Can you work these out from the model? Positions are in its coordinate system, mm. A direction names the side the tool comes from. Coordinates: 2 decimals unless noted, no trailing zeros. Order: outer loops, then holes, each group sorted by start corner. A loop starts at its lowest first (then second) coordinate and runs counter-clockwise, first axis right, second up. Notation, with made-up numbers: (47.5, 88.5) -> (100.5, 88.5) arc R26 ccw to (100.5, 107.5) -> close; hole circle Ø10 at (40.25, 72). An arc over 180 degrees is marked (long way). Write item = value, one per line.
```python
from build123d import *

# Parameters (mm, degrees)
SKETCH_1_W          = 200
SKETCH_1_H          = 400
EXTRUDE_1_DEPTH     = 8
SKETCH_2_R          = 30
CUT_EXTRUDE_1_DEPTH = 10
SKETCH_3_R          = 2.25
CUT_EXTRUDE_2_DEPTH = 10
SKETCH_4_R          = 4
CUT_EXTRUDE_3_DEPTH = 4.4
FILLET_1_R          = 60
SKETCH_5_R          = 4.25
CUT_EXTRUDE_4_DEPTH = 10
SKETCH_6_W          = 50
SKETCH_6_H          = 220
CUT_EXTRUDE_5_DEPTH = 10
FILLET_2_R          = 10
SKETCH_7_W          = 100
SKETCH_7_H          = 120
CUT_EXTRUDE_6_DEPTH = 84
FILLET_3_R          = 10


with BuildPart() as part:
    # 草图1 → 凸台-拉伸1 (new body)
    with BuildSketch(Plane.XY):
        with Locations((0, 200)):
            Rectangle(SKETCH_1_W, SKETCH_1_H)
    extrude(amount=EXTRUDE_1_DEPTH)

    # 草图2 → 切除-拉伸1 (cut)
    with BuildSketch(Plane(origin=(0, 0, 0), x_dir=(-1, 0, 0), z_dir=(0, 0, -1))):
        with Locations((0, 300)):
            Circle(SKETCH_2_R)
    extrude(amount=-CUT_EXTRUDE_1_DEPTH, mode=Mode.SUBTRACT)

    # 草图3 → 切除-拉伸2 (cut)
    with BuildSketch(Plane(origin=(0, 0, 0), x_dir=(-1, 0, 0), z_dir=(0, 0, -1))):
        with Locations((0, 341.5)):
            Circle(SKETCH_3_R)
        with Locations((29.344931419, 329.344931419)):
            Circle(SKETCH_3_R)
        with Locations((41.5, 300)):
            Circle(SKETCH_3_R)
        with Locations((29.344931419, 270.655068581)):
            Circle(SKETCH_3_R)
        with Locations((0, 258.5)):
            Circle(SKETCH_3_R)
        with Locations((-29.344931419, 270.655068581)):
            Circle(SKETCH_3_R)
        with Locations((-41.5, 300)):
            Circle(SKETCH_3_R)
        with Locations((-29.344931419, 329.344931419)):
            Circle(SKETCH_3_R)
    extrude(amount=-CUT_EXTRUDE_2_DEPTH, mode=Mode.SUBTRACT)

    # 草图4 → 切除-拉伸3 (cut)
    with BuildSketch(Plane.XY.offset(8)):
        with Locations((29.344931419, 329.344931419)):
            Circle(SKETCH_4_R)
        with Locations((41.5, 300)):
            Circle(SKETCH_4_R)
        with Locations((29.344931419, 270.655068581)):
            Circle(SKETCH_4_R)
        with Locations((0, 258.5)):
            Circle(SKETCH_4_R)
        with Locations((-29.344931419, 270.655068581)):
            Circle(SKETCH_4_R)
        with Locations((-41.5, 300)):
            Circle(SKETCH_4_R)
        with Locations((-29.344931419, 329.344931419)):
            Circle(SKETCH_4_R)
        with Locations((0, 341.5)):
            Circle(SKETCH_4_R)
    extrude(amount=-CUT_EXTRUDE_3_DEPTH, mode=Mode.SUBTRACT)

    # 圆角1
    fillet_1_edges = [part.edges().sort_by_distance(p)[0] for p in [
        (100, 400, 4),
        (-100, 400, 4),
    ]]
    fillet(fillet_1_edges, radius=FILLET_1_R)

    # 草图5 → 切除-拉伸4 (cut)
    with BuildSketch(Plane(origin=(0, 0, 0), x_dir=(-1, 0, 0), z_dir=(0, 0, -1))):
        with Locations((-15, 25)):
            Circle(SKETCH_5_R)
        with Locations((15, 25)):
            Circle(SKETCH_5_R)
        with Locations((-15, 65)):
            Circle(SKETCH_5_R)
        with Locations((15, 65)):
            Circle(SKETCH_5_R)
        with Locations((-15, 175)):
            Circle(SKETCH_5_R)
        with Locations((-15, 135)):
            Circle(SKETCH_5_R)
        with Locations((15, 135)):
            Circle(SKETCH_5_R)
        with Locations((15, 175)):
            Circle(SKETCH_5_R)
    extrude(amount=-CUT_EXTRUDE_4_DEPTH, mode=Mode.SUBTRACT)

    # 草图6 → 切除-拉伸5 (cut)
    with BuildSketch(Plane.XY.offset(8)):
        with Locations((-75, 110)):
            Rectangle(SKETCH_6_W, SKETCH_6_H)
        with Locations((75, 110)):
            Rectangle(SKETCH_6_W, SKETCH_6_H)
    extrude(amount=-CUT_EXTRUDE_5_DEPTH, mode=Mode.SUBTRACT)

    # 圆角2
    fillet_2_edges = [part.edges().sort_by_distance(p)[0] for p in [
        (100, 220, 4),
        (50, 220, 4),
        (-100, 220, 4),
        (-50, 220, 4),
    ]]
    fillet(fillet_2_edges, radius=FILLET_2_R)

    # 草图7 → 切除-拉伸6 (cut)
    with BuildSketch(Plane(origin=(0, 0, 0), x_dir=(-1, 0, 0), z_dir=(0, 0, -1))):
        with Locations((0, 60)):
            Rectangle(SKETCH_7_W, SKETCH_7_H)
    extrude(amount=-CUT_EXTRUDE_6_DEPTH, mode=Mode.SUBTRACT)

    # 圆角3
    fillet_3_edges = [part.edges().sort_by_distance(p)[0] for p in [
        (50, 120, 4),
        (-50, 120, 4),
    ]]
    fillet(fillet_3_edges, radius=FILLET_3_R)


solid = part.part
```
Item 1: For faces 1 (the flat face through (-75, 220, 4)), 2 (the cylindrical face through (-14.447, 179.214, 3.944)), 3 (the cylindrical face through (-27.499, 267.106, 5.831)), which set-ups out of +Z, -Z, +X, -X, +Y, -Y let a thin tool reach every point of the face, with its end or its side?
A:
face_1 = +Z, -Z, -X, -Y
face_2 = +Z, -Z
face_3 = +Z
Item 2: I want a section at A-A, the plane y = 175. Please give me the cut outline in (x, z).
A:
outline = (-50, 0) -> (-19.25, 0) -> (-19.25, 8) -> (-50, 8) -> close; (-10.75, 0) -> (10.75, 0) -> (10.75, 8) -> (-10.75, 8) -> close; (19.25, 0) -> (50, 0) -> (50, 8) -> (19.25, 8) -> close
Item 3: I want a section at B-B, the plane z = 2. Give the number of separate pieces and of enclosed holes in the cut face, plus the area to 3 significant figures.
A:
separate_pieces = 1
enclosed_holes = 13
area = 41,200 mm2
Item 4: I want a section at D-D, the plane y = 369. Please give me the cut outline in (x, z), plus the area to 3 significant figures.
A:
outline = (-92.53, 0) -> (92.53, 0) -> (92.53, 8) -> (-92.53, 8) -> close
area = 1,480 mm2
Item 5: I'm going to push flat-ended pins straight in: P1, Ø6.5, axis at x = 29.34, y = 270.66, coming from the +Z side; P2, Ø1.5, axis at y = 205.5, z = 6.5, coming from the +X side; P3, Ø7, axis at x = 15, y = 175, coming from the -Z side. Where does each tip first touch, or does it pass through?
A:
P1 = 3.6
P2 = 50
P3 = through
Item 6: If I drill on probe 1 along Y at (x, z) = (0, 5.25); probe 2 along X at (y, z) = (258.5, 7); probe 3 along X at (y, z) = (341.5, 2.8), over which ranges is the centre line in solid material (lowest first)?
A:
probe_1 = 120 to 254.5, 262.5 to 270, 330 to 337.5, 345.5 to 400
probe_2 = -100 to -4, 4 to 100
probe_3 = -99.98 to -2.25, 2.25 to 99.98
Item 7: I want a section at C-C, the plane x = 79. Please give me the cut outline in (y, z), plus the area to 3 significant figures.
A:
outline = (220, 0) -> (385.6, 0) -> (385.6, 8) -> (220, 8) -> close
area = 1,320 mm2
Item 8: If we mould it in two halves opening along Y, with no side actions, what happens to faces 4 (the cylindrical face through (31.2, 325.8, 5.8)), 5 (the flat face through (-1, 400, 4)), 6 (the flat face through (75, 220, 4))? For each: pulls with the +Y half, pulls with the -Y half, needs draft (parallel to the pull), parting line crosses it, or undercut.
A:
face_4 = undercut
face_5 = pulls with the +Y half
face_6 = pulls with the -Y half
